from build123d import *

# Parameters (mm, degrees)
SKETCH1_W           = 143
SKETCH1_H           = 68
BOSS_EXTRUDE1_DEPTH = 17
FILLET1_R           = 7
FILLET2_R           = 7


with BuildPart() as part:
    # Sketch1 → Boss-Extrude1 (new body)
    with BuildSketch(Plane.XY):
        with Locations((-65.703539823, 13.690265487)):
            Rectangle(SKETCH1_W, SKETCH1_H)
    extrude(amount=BOSS_EXTRUDE1_DEPTH)

    # Fillet1
    fillet1_edges = [part.edges().sort_by_distance(p)[0] for p in [
        (5.796460177, 13.690265487, 17),
        (-65.703539823, 47.690265487, 17),
        (-137.203539823, 13.690265487, 17),
        (-65.703539823, 47.690265487, 0),
        (5.796460177, 13.690265487, 0),
        (-65.703539823, -20.309734513, 0),
        (-137.203539823, 13.690265487, 0),
        (-137.203539823, 47.690265487, 8.5),
        (5.796460177, 47.690265487, 8.5),
        (-65.703539823, -20.309734513, 17),
    ]]
    fillet(fillet1_edges, radius=FILLET1_R)

    # Fillet2
    # the kernel refuses this fillet: 7 mm, written as the material it takes off along each edge
    with BuildSketch(Plane(origin=(-130.203539823, -13.309734513, 10), x_dir=(0, -1, 0), z_dir=(-1, 0, 0))) as fillet2_piece_1_section:
        Polygon((0, 0), (FILLET2_R, 0), (FILLET2_R, FILLET2_R), (0, FILLET2_R), align=None)
    fillet2_piece_1 = extrude(amount=FILLET2_R, mode=Mode.PRIVATE)
    fillet2_piece_1 = fillet2_piece_1 - Plane(origin=(-130.203539823, -13.309734513, 10), x_dir=(0, 0.7071067811865475, -0.7071067811865475), z_dir=(-1, 0, 0)) * Sphere(FILLET2_R, mode=Mode.PRIVATE)
    add(fillet2_piece_1, mode=Mode.SUBTRACT)
    with BuildSketch(Plane(origin=(-130.203539823, -13.309734513, 7), x_dir=(0, -1, 0), z_dir=(-1, 0, 0))) as fillet2_piece_2_section:
        Polygon((0, 0), (FILLET2_R, 0), (FILLET2_R, -FILLET2_R), (0, -FILLET2_R), align=None)
    fillet2_piece_2 = extrude(amount=FILLET2_R, mode=Mode.PRIVATE)
    fillet2_piece_2 = fillet2_piece_2 - Plane(origin=(-130.203539823, -13.309734513, 7), x_dir=(0, 0.7071067811865475, 0.7071067811865475), z_dir=(-1, 0, 0)) * Sphere(FILLET2_R, mode=Mode.PRIVATE)
    add(fillet2_piece_2, mode=Mode.SUBTRACT)
    with BuildSketch(Plane(origin=(-1.203539823, -13.309734513, 10), x_dir=(0, -1, 0), z_dir=(1, 0, 0))) as fillet2_piece_3_section:
        Polygon((0, 0), (FILLET2_R, 0), (FILLET2_R, -FILLET2_R), (0, -FILLET2_R), align=None)
    fillet2_piece_3 = extrude(amount=FILLET2_R, mode=Mode.PRIVATE)
    fillet2_piece_3 = fillet2_piece_3 - Plane(origin=(-1.203539823, -13.309734513, 10), x_dir=(0, 0.7071067811865475, -0.7071067811865475), z_dir=(1, 0, 0)) * Sphere(FILLET2_R, mode=Mode.PRIVATE)
    add(fillet2_piece_3, mode=Mode.SUBTRACT)
    with BuildSketch(Plane(origin=(-1.203539823, -13.309734513, 7), x_dir=(0, -1, 0), z_dir=(1, 0, 0))) as fillet2_piece_4_section:
        Polygon((0, 0), (FILLET2_R, 0), (FILLET2_R, FILLET2_R), (0, FILLET2_R), align=None)
    fillet2_piece_4 = extrude(amount=FILLET2_R, mode=Mode.PRIVATE)
    fillet2_piece_4 = fillet2_piece_4 - Plane(origin=(-1.203539823, -13.309734513, 7), x_dir=(0, 0.7071067811865475, 0.7071067811865475), z_dir=(1, 0, 0)) * Sphere(FILLET2_R, mode=Mode.PRIVATE)
    add(fillet2_piece_4, mode=Mode.SUBTRACT)
    with BuildSketch(Plane(origin=(5.796460177, -20.309734513, 7), x_dir=(0, 1, 0), z_dir=(0, 0, 1))) as fillet2_piece_5:
        with BuildLine():
            CenterArc((FILLET2_R, FILLET2_R), FILLET2_R, 180, 90)
            Line((0, FILLET2_R), (0, 0))
            Line((0, 0), (FILLET2_R, 0))
        make_face()
    extrude(amount=3, mode=Mode.SUBTRACT)
    with BuildSketch(Plane(origin=(-137.203539823, -20.309734513, 7), x_dir=(0, 1, 0), z_dir=(0, 0, 1))) as fillet2_piece_6:
        with BuildLine():
            CenterArc((FILLET2_R, -FILLET2_R), FILLET2_R, 90, 90)
            Line((0, -FILLET2_R), (0, 0))
            Line((0, 0), (FILLET2_R, 0))
        make_face()
    extrude(amount=3, mode=Mode.SUBTRACT)


solid = part.part
Read the model definition and answer for the solid it produces. Units are mm, in the model's axes. Round coordinates to 2 decimals unless told otherwise and drop trailing zeros. Write each loop counter-clockwise with the first axis right and the second up, starting at its lowest first coordinate (ties: lowest second). Pieces come first, ordered by that corner, then holes. Notation, with made-up numbers: (56, 10) - (104, 10) arc R34 cw to (104, 46) - close; hole circle Ø9 at (74.5, 80). An arc over 180 degrees is marked (long way). Use a Markdown table: item, result.
(1) Straight lines are drawn through the part: line 1 along Y through (x, z) = (-32, 6.75); line 2 along X through (y, z) = (12, 6.75); line 3 along X through (y, z) = (33, 1). For each, find the intervals that lie inside material, in ascending order. Write a range as [from, to].
Reported:
| item | result |
|---|---|
| line 1 | [-20.31, 47.69] |
| line 2 | [-137.2, 5.79] |
| line 3 | [-133.81, 2.4] |
(2) The part is cut by section B-B (y = 7). Write down the section's boundary in (x, z).
Reported:
| item | result |
|---|---|
| outline | (-137.2, 7) arc R7 ccw to (-130.2, 0) - (-1.2, 0) arc R7 ccw to (5.8, 7) - (5.8, 10) arc R7 ccw to (-1.2, 17) - (-130.2, 17) arc R7 ccw to (-137.2, 10) - close |
(3) Each of these flat-tipped pins is pushed along its axis until it touches: pin 1 Ø4 at (x, z) = (-22, 4) entering from -Y; pin 2 Ø1 at (y, z) = (38.5, 12) entering from +X; pin 3 Ø6 at (x, z) = (-29.5, 15) entering from -Y. Where does it stop, or does it pass through?
Reported:
| item | result |
|---|---|
| pin 1 | y = -20.24 |
| pin 2 | x = 5.63 |
| pin 3 | y = -20.02 |
(4) The part is cut by section A-A (x = -66). Write down the section's boundary in (y, z), then the cut area to 3 significant figures.
Reported:
| item | result |
|---|---|
| outline | (-20.31, 7) arc R7 ccw to (-13.31, 0) - (40.69, 0) arc R7 ccw to (47.69, 7) - (47.69, 10) arc R7 ccw to (40.69, 17) - (-13.31, 17) arc R7 ccw to (-20.31, 10) - close |
| area | 1,110 mm2 |
